Can you work these out from the model? Positions are in its coordinate system, mm. A direction names the side the tool comes from. Give positions to 0.01 mm unless a question says otherwise; leave off trailing zeros. Order: outer loops, then holes, each group sorted by start corner. A loop starts at its lowest first (then second) coordinate and runs counter-clockwise, first axis right, second up.
Item 1: I want a section at A-A, the plane x = -15.5. Write out the boundary of the cut face in (y, z) (1 decimal), then the cut area to 3 significant figures.
Item 2: If we mould it in two halves opening along Z, with no side actions, what happens to faces 4 (the flat face through (0, -2, 9)), 5 (the flat face through (-10, -2, 0)), 6 (the flat face through (-8.284, -2.392, 8.384)), 7 (the flat face through (-4.762, -2, 2))? For each: +Z half, -Z half, draft (parallel to the pull), parting line (faces both ways), or undercut.
Item 3: I want a section at D-D, the plane z = 7.25. Write out the boundary of the cut face in (x, y) (1 decimal), then the cut area to 3 significant figures.
Item 4: If I drill on line 1 along Z through (x, y) = (-11, -0.9); line 2 along X through (y, z) = (-0.25, 5.25); line 3 along Z through (x, y) = (-10.25, -2.2), over which ranges is the centre line in solid material (lowest first)?
Item 5: I want a section at C-C, the plane y = -1.3. Write out the boundary of the cut face in (x, z).
Item 6: I'm going to push flat-ended pins straight in: pin 1 Ø0.5 at (y, z) = (-2.5, 2) entering from -X; pin 2 Ø1 at (x, y) = (-10, -2.5) entering from +Z; pin 3 Ø1.4 at (x, y) = (-2, -1.5) entering from +Z. Where does each tip first touch, or does it pass through?
Item 7: Which directions (+Z, -Z, +X, -X, +Y, -Y) give clear straight access to the entire face, cutting with the end or side of a thin tool? Please do faces 1 (the flat face through (-1.53, -2, 10)), 2 (the flat face through (-11, -2, 1.53)), 3 (the flat face through (-4.762, -1, 14)).
Item 8: I want a section at B-B, the plane z = 4.25. Write out the boundary of the cut face in (x, y) (3 decimals), then the cut area to 3 significant figures.
```python
from build123d import *

# Parameters (mm, degrees)
F0_W     = 1.53035
F0_H     = 11.1125
F0_H_2   = 3.175
F0_W_2   = 1.7018
F0_H_3   = 1.53035
F0_W_3   = 11.1125
F0_W_4   = 3.175
F0_H_4   = 1.7018
F1_DEPTH = 3.175
F3_DEPTH = 1.5875
F4_SIZE  = 0.79375
F5_DEPTH = 6.35
F6_DEPTH = 3.175


with BuildPart() as f1:
    # F0 (on Front) → F1 (new body)
    with BuildSketch(Plane.XZ):
        with Locations((-0.765175, 13.49375)):
            Rectangle(F0_W, F0_H)
        with Locations((-3.997325, 13.49375)):
            Rectangle(F0_W, F0_H)
        with Locations((-0.765175, 6.35)):
            Rectangle(F0_W, F0_H_2)
        with Locations((-2.38125, 6.35)):
            Rectangle(F0_W_2, F0_H_2)
        with Locations((-3.997325, 6.35)):
            Rectangle(F0_W, F0_H_2)
        Polygon((-4.7625, 0), (0, 0), (0, 4.7625), (-1.53035, 4.7625), (-1.53035, 1.53035), (-4.7625, 1.53035), align=None)
        Polygon((-4.7625, 3.23215), (-4.7625, 1.53035), (-1.53035, 1.53035), (-1.53035, 4.7625), (-3.23215, 4.7625), (-3.23215, 3.23215), align=None)
        with Locations((-3.997325, 3.997325)):
            Rectangle(F0_W, F0_H_3)
        with Locations((-13.49375, 3.997325)):
            Rectangle(F0_W_3, F0_H_3)
        with Locations((-13.49375, 0.765175)):
            Rectangle(F0_W_3, F0_H_3)
        with Locations((-6.35, 0.765175)):
            Rectangle(F0_W_4, F0_H_3)
        with Locations((-6.35, 2.38125)):
            Rectangle(F0_W_4, F0_H_4)
        with Locations((-6.35, 3.997325)):
            Rectangle(F0_W_4, F0_H_3)
    extrude(amount=F1_DEPTH)

    # F2 (on face) → F3 (join)
    with BuildSketch(Plane.XZ.offset(3.175)):
        Polygon((-4.7625, 11.90625), (-11.90625, 4.7625), (-4.7625, 4.7625), align=None)
    extrude(amount=-F3_DEPTH)

    # F4
    f4_edges = [f1.edges().sort_by_distance(p)[0] for p in [
        (-19.05, -1.5875, 3.23215),
        (-19.05, -1.5875, 1.53035),
        (-1.53035, -1.5875, 19.05),
        (-3.23215, -1.5875, 19.05),
    ]]
    chamfer(f4_edges, length=F4_SIZE)

    # F5 (cut): a face of the model
    f5_faces = [f1.faces().sort_by_distance(p)[0] for p in [
        (-2.38125, -1.5875, 7.9375),
    ]]
    extrude(f5_faces, amount=-F5_DEPTH, mode=Mode.SUBTRACT)

    # F6 (cut): a face of the model
    f6_faces = [f1.faces().sort_by_distance(p)[0] for p in [
        (-7.9375, -1.5875, 2.38125),
    ]]
    extrude(f6_faces, amount=-F6_DEPTH, mode=Mode.SUBTRACT)


solid = f1.part
```
Results list:
1. outline: (-3.2, 0) - (0, 0) - (0, 1.5) - (-3.2, 1.5) - close; (-3.2, 3.2) - (0, 3.2) - (0, 4.8) - (-3.2, 4.8) - close
1. area: 9.72 mm2
2. face 4: draft
2. face 5: -Z half
2. face 6: +Z half
2. face 7: undercut
3. outline: (-9.4, -3.2) - (-3.2, -3.2) - (-3.2, 0) - (-4.8, 0) - (-4.8, -1.6) - (-9.4, -1.6) - close; (-1.5, -3.2) - (0, -3.2) - (0, 0) - (-1.5, 0) - close
3. area: 17.1 mm2
4. line 1: z = 0 to 1.53, 3.23 to 4.76
4. line 2: x = -4.76 to -3.23, -1.53 to 0
4. line 3: z = 0 to 1.53, 3.23 to 6.42
5. outline: (-19.05, 0) - (0, 0) - (0, 19.05) - (-0.74, 19.05) - (-1.53, 18.26) - (-1.53, 1.59) - (-3.23, 1.59) - (-3.23, 18.26) - (-4.03, 19.05) - (-4.76, 19.05) - (-4.76, 4.76) - (-19.05, 4.76) - (-19.05, 4.03) - (-18.26, 3.23) - (-4.76, 3.23) - (-4.76, 1.53) - (-18.26, 1.53) - (-19.05, 0.74) - close
6. pin 1: stops at x = -4.76
6. pin 2: stops at z = 7.17
6. pin 3: stops at z = 18.49
7. face 1: +Z, +Y, -Y
7. face 2: -X, +Y, -Y
7. face 3: +Z, -X, +Y
8. outline: (-19.05, -3.175) - (-3.232, -3.175) - (-3.232, 0) - (-19.05, 0) - close; (-1.53, -3.175) - (0, -3.175) - (0, 0) - (-1.53, 0) - close
8. area: 55.1 mm2
